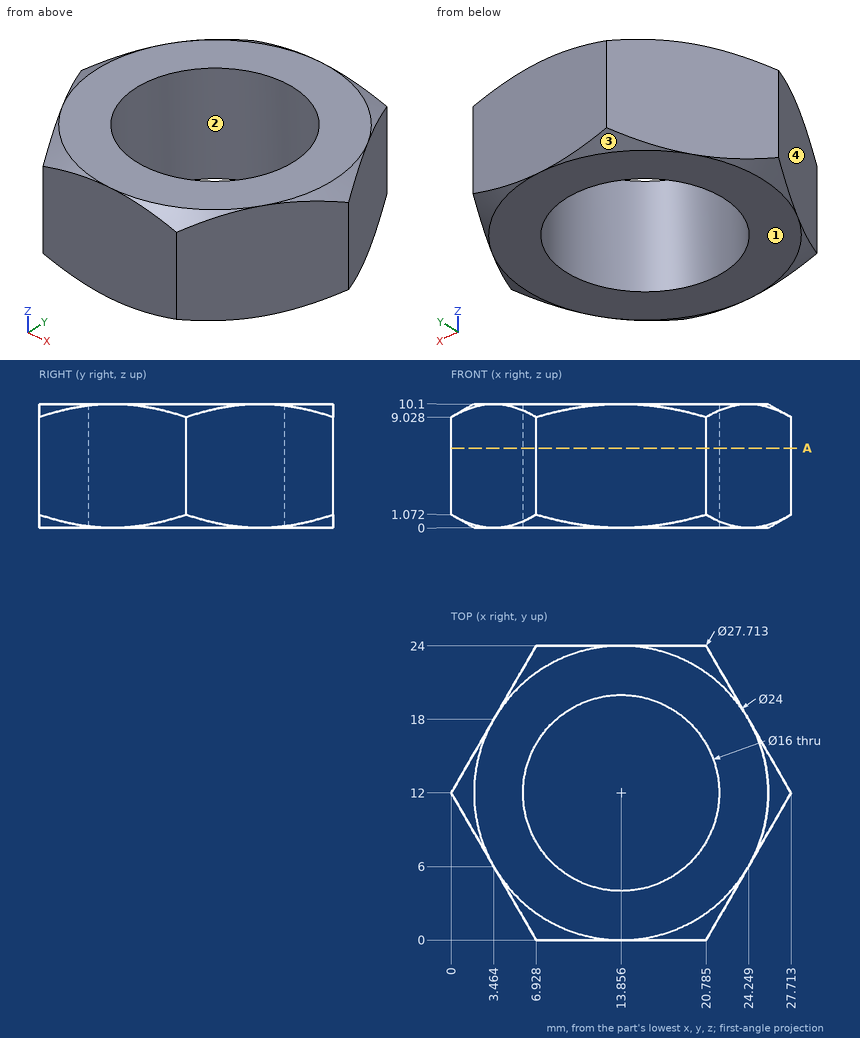
Source: three-view drawing plus pictorial views. Frame: mm from the lowest corner of the part. Round coordinates to 2 decimals unless told otherwise and drop trailing zeros. Loops run counter-clockwise (first coordinate to the right, second up) from the corner with the lowest first, then second, coordinate; pieces in that order, holes last.
Q1. Mould query, pull axis Y, two halves, no side actions, for the marked faces 1, 2, 3 and 4. Classes: pulls with the +Y half, pulls with the -Y half, needs draft (parallel to the pull), parting line crosses it, or undercut.
Q2. Ray query, line 1 (Y direction, x = 14, z = 6.75); line 2 (X direction, y = 6.75, z = 7.25) (1 decimal); line 3 (Y direction, x = 7.5, z = 8.25) (1 decimal). Return the intervals inside material, ascending.
Q3. Section A-A, the plane z = 6.5. Return loops of the section in (x, y) (1 decimal), plus the area to 3 significant figures.
Q4. First-contact query: P1, Ø3, axis at y = 19, z = 2.5, coming from the -X side (1 decimal); P2, Ø12, axis at x = 14.5, y = 13.5, coming from the +Z side; P3, Ø5, axis at y = 7, z = 6, coming from the +X side; P4, Ø6, axis at y = 4, z = 7, coming from the -X side. Flat tips, straight axial feed; report the tip coordinate or a pass-through.
Solutions:
1. face 1: needs draft
1. face 2: undercut
1. face 3: pulls with the +Y half
1. face 4: pulls with the -Y half
2. line 1: y = 0 to 4, 20 to 24
2. line 2: x = 3 to 7.8, 19.9 to 24.7
2. line 3: y = 0 to 7.1, 16.9 to 24
3. outline: (0, 12) - (6.9, 0) - (20.8, 0) - (27.7, 12) - (20.8, 24) - (6.9, 24) - close; hole circle Ø16 at (13.9, 12)
3. area: 298 mm2
4. P1: stops at x = 3.2
4. P2: passes through
4. P3: stops at x = 26.27
4. P4: stops at x = 2.89
